Geometry check sheet. Reference: the model listing, model coordinates, mm. Face numbers are marked on the shaded views. A direction names the side the tool comes from. Give positions to 0.01 mm unless a question says otherwise; leave off trailing zeros. Loops run counter-clockwise (first coordinate to the right, second up) from the corner with the lowest first, then second, coordinate; pieces in that order, holes last.
1. Release check for a two-part mould opening along Z. For the marked faces 3, 4, 5 and 6 record: +Z half, -Z half, draft (parallel to the pull), parting line (faces both ways), or undercut.
2. Cross-section at C-C, the plane x = 45. Record the cut outline in (y, z).
3. Tool access check on the marked faces 1 and 2. Record the directions out of +Z, -Z, +X, -X, +Y, -Y that give a thin tool (end or side, any length) a straight path to the whole face; none if there is none.
4. Go/stop test with flat-tipped pins: pin 1 Ø3 at (x, z) = (14.5, -34.5) entering from -Y; pin 2 Ø5 at (x, z) = (0, -21.5) entering from +Y; pin 3 Ø0.8 at (x, z) = (22.5, 21.5) entering from +Y; pin 4 Ø2.5 at (x, z) = (-26, -2.5) entering from +Y. Record where each tip stops, or that it passes through.
5. Cross-section at A-A, the plane y = 10. Record the cut outline in (x, z).
6. Cross-section at D-D, the plane y = 23. Record the cut outline in (x, z), plus the area to 4 significant figures.
7. Material ranges on L1, parallel to X at y = 7.5, z = 0; L2, parallel to Z at x = 33, y = 33.5; L3, parallel to Z at x = -30, y = 29.5, recorded low to high.
8. Cross-section at B-B, the plane x = 31. Record the cut outline in (y, z).
from build123d import *

# Parameters (mm, degrees)
SKETCH1_W               = 87
SKETCH1_H               = 60
HOUSING_DEPTH           = 35
SKETCH4_W               = 82
SKETCH4_H               = 55
HOUSEINTERNALCUT_DEPTH  = 30
SKETCH6_W               = 3.7
SKETCH6_H               = 8.5
SWITCHEXTERNALCUT_DEPTH = 2
SKETCH8_W               = 1.7
SKETCH8_H               = 3.6
SWITCHINTERNALCUT_DEPTH = 4
SKETCH10_R              = 6
BUZZEREXTERNALCUT_DEPTH = 2
SKETCH12_R              = 0.35
BUZZERINTERNALCUT_DEPTH = 4
SKETCH14_W              = 4.6
SKETCH14_H              = 6.1
BUTTONEXTERNALCUT_DEPTH = 2
SKETCH16_R              = 1.5
BUTTONINTERNALCUT_DEPTH = 4
SKETCH29_R              = 17.515
WICHARGECUT_DEPTH       = 3.5
SKETCH30_W              = 59
SKETCH30_H              = 39
RFIDMODULECUT_DEPTH     = 1
SKETCH32_W              = 71
SKETCH32_H              = 25
DISPLAYCUT_DEPTH        = 3.5
MICROUSBCUT_DEPTH       = 2.5
SKETCH34_W              = 6.5
SKETCH34_H              = 3
CLIPSCUT_DEPTH          = 88
SKETCH35_R              = 0.45
RESETCUT_DEPTH          = 6


with BuildPart() as part:
    # Sketch1 → Housing (new body)
    with BuildSketch(Plane(origin=(0, 0, 0), x_dir=(1, 0, 0), z_dir=(0, 1, 0))):
        with Locations((6.529661017, 6.430084746)):
            Rectangle(SKETCH1_W, SKETCH1_H)
    extrude(amount=HOUSING_DEPTH)

    # Sketch4 → HouseInternalCut (cut)
    with BuildSketch(Plane(origin=(0, 35, 0), x_dir=(1, 0, 0), z_dir=(0, 1, 0))):
        with Locations((6.529661017, 6.430084746)):
            Rectangle(SKETCH4_W, SKETCH4_H)
    extrude(amount=-HOUSEINTERNALCUT_DEPTH, mode=Mode.SUBTRACT)

    # Sketch6 → SwitchExternalCut (cut)
    with BuildSketch(Plane(origin=(-29.459679841, 5, 17.678662656), x_dir=(1, 0, 0), z_dir=(0, 1, 0))):
        with Locations((4.354897879, 7.989454328)):
            Rectangle(SKETCH6_W, SKETCH6_H)
    extrude(amount=-SWITCHEXTERNALCUT_DEPTH, mode=Mode.SUBTRACT)

    # Sketch8 → SwitchInternalCut (cut, through all)
    with BuildSketch(Plane(origin=(-29.459679841, 3, 17.678662656), x_dir=(1, 0, 0), z_dir=(0, 1, 0))):
        with Locations((4.354897879, 7.989454328)):
            Rectangle(SKETCH8_W, SKETCH8_H)
    extrude(amount=-SWITCHINTERNALCUT_DEPTH, mode=Mode.SUBTRACT)

    # Sketch10 → BuzzerExternalCut (cut)
    with BuildSketch(Plane(origin=(-0.314920006, 5, -24.188639302), x_dir=(1, 0, 0), z_dir=(0, 1, 0))):
        with Locations((-25.006618322, 0)):
            Circle(SKETCH10_R)
    extrude(amount=-BUZZEREXTERNALCUT_DEPTH, mode=Mode.SUBTRACT)

    # Sketch12 → BuzzerInternalCut (cut, through all)
    with BuildSketch(Plane(origin=(-0.314920006, 3, -24.188639302), x_dir=(1, 0, 0), z_dir=(0, 1, 0))):
        with Locations((-24.042348329, 4.522315504)):
            Circle(SKETCH12_R)
        with Locations((-26.042348329, 3.020429056)):
            Circle(SKETCH12_R)
        with Locations((-28.042348329, 3.020429056)):
            Circle(SKETCH12_R)
        with Locations((-30.042348329, 1.518542609)):
            Circle(SKETCH12_R)
        with Locations((-30.042348329, 0.016656161)):
            Circle(SKETCH12_R)
        with Locations((-30.042348329, -1.485230286)):
            Circle(SKETCH12_R)
        with Locations((-28.042348329, 0.016656161)):
            Circle(SKETCH12_R)
        with Locations((-28.042348329, 1.518542609)):
            Circle(SKETCH12_R)
        with Locations((-28.042348329, -1.485230286)):
            Circle(SKETCH12_R)
        with Locations((-28.042348329, -2.987116733)):
            Circle(SKETCH12_R)
        with Locations((-26.042348329, 0.016656161)):
            Circle(SKETCH12_R)
        with Locations((-26.042348329, 1.518542609)):
            Circle(SKETCH12_R)
        with Locations((-26.042348329, -1.485230286)):
            Circle(SKETCH12_R)
        with Locations((-26.042348329, -2.987116733)):
            Circle(SKETCH12_R)
        with Locations((-26.042348329, -4.489003181)):
            Circle(SKETCH12_R)
        with Locations((-24.042348329, -4.489003181)):
            Circle(SKETCH12_R)
        with Locations((-24.042348329, -2.987116733)):
            Circle(SKETCH12_R)
        with Locations((-24.042348329, -1.485230286)):
            Circle(SKETCH12_R)
        with Locations((-24.042348329, 0.016656161)):
            Circle(SKETCH12_R)
        with Locations((-24.042348329, 1.518542609)):
            Circle(SKETCH12_R)
        with Locations((-24.042348329, 3.020429056)):
            Circle(SKETCH12_R)
        with Locations((-22.042348329, 3.020429056)):
            Circle(SKETCH12_R)
        with Locations((-22.042348329, 1.518542609)):
            Circle(SKETCH12_R)
        with Locations((-22.042348329, 0.016656161)):
            Circle(SKETCH12_R)
        with Locations((-22.042348329, -1.485230286)):
            Circle(SKETCH12_R)
        with Locations((-22.042348329, -2.987116733)):
            Circle(SKETCH12_R)
        with Locations((-20.042348329, -1.485230286)):
            Circle(SKETCH12_R)
        with Locations((-20.042348329, 0.016656161)):
            Circle(SKETCH12_R)
        with Locations((-20.042348329, 1.518542609)):
            Circle(SKETCH12_R)
        with Locations((-26.042348329, 4.522315504)):
            Circle(SKETCH12_R)
    extrude(amount=-BUZZERINTERNALCUT_DEPTH, mode=Mode.SUBTRACT)

    # Sketch14 → ButtonExternalCut (cut)
    with BuildSketch(Plane(origin=(-24.227687265, 5, -14.72402786), x_dir=(1, 0, 0), z_dir=(0, 1, 0))):
        with Locations((-1.096336387, -10.602688636)):
            Rectangle(SKETCH14_W, SKETCH14_H)
    extrude(amount=-BUTTONEXTERNALCUT_DEPTH, mode=Mode.SUBTRACT)

    # Sketch16 → ButtonInternalCut (cut, through all)
    with BuildSketch(Plane(origin=(-24.227687265, 3, -14.72402786), x_dir=(1, 0, 0), z_dir=(0, 1, 0))):
        with Locations((-1.096336387, -10.602688636)):
            Circle(SKETCH16_R)
    extrude(amount=-BUTTONINTERNALCUT_DEPTH, mode=Mode.SUBTRACT)

    # Sketch29 → WiChargeCut (cut)
    with BuildSketch(Plane(origin=(0, 5, 0), x_dir=(1, 0, 0), z_dir=(0, 1, 0))):
        with Locations((6.529661017, 6.430084746)):
            Circle(SKETCH29_R)
    extrude(amount=-WICHARGECUT_DEPTH, mode=Mode.SUBTRACT)

    # Sketch30 → RFIDModuleCut (cut)
    with BuildSketch(Plane(origin=(0, 0, 21.069915254), x_dir=(-1, 0, 0), z_dir=(0, 0, -1))):
        with Locations((-10.029661017, 25.5)):
            Rectangle(SKETCH30_W, SKETCH30_H)
    extrude(amount=-RFIDMODULECUT_DEPTH, mode=Mode.SUBTRACT)

    # Sketch32 → DisplayCut (cut, through all)
    with BuildSketch(Plane.XY.offset(-33.930084746)):
        with Locations((6.529661017, 20.5)):
            Rectangle(SKETCH32_W, SKETCH32_H)
    extrude(amount=-DISPLAYCUT_DEPTH, mode=Mode.SUBTRACT)

    # Sketch33 → MicroUSBCut (cut)
    with BuildSketch(Plane(origin=(50.029661017, 0, 0), x_dir=(0, 0, -1), z_dir=(1, 0, 0))):
        with BuildLine():
            Line((2.705084746, 11), (10.155084746, 11))
            ThreePointArc((10.155084746, 11), (11.155084746, 10), (10.155084746, 9))
            Line((10.155084746, 9), (2.705084746, 9))
            ThreePointArc((2.705084746, 9), (1.705084746, 10), (2.705084746, 11))
        make_face()
    extrude(amount=-MICROUSBCUT_DEPTH, mode=Mode.SUBTRACT)

    # Sketch34 → ClipsCut (cut, through all)
    with BuildSketch(Plane.ZY.offset(36.970338983)):
        with Locations((-22.680084746, 28.64745115)):
            Rectangle(SKETCH34_W, SKETCH34_H)
        with Locations((9.819915254, 28.64745115)):
            Rectangle(SKETCH34_W, SKETCH34_H)
    extrude(amount=-CLIPSCUT_DEPTH, mode=Mode.SUBTRACT)

    # Sketch35 → ResetCut (cut, through all)
    with BuildSketch(Plane(origin=(0, 5, 0), x_dir=(1, 0, 0), z_dir=(0, 1, 0))):
        with Locations((46.529661017, -2.509915254)):
            Circle(SKETCH35_R)
    extrude(amount=-RESETCUT_DEPTH, mode=Mode.SUBTRACT)


solid = part.part
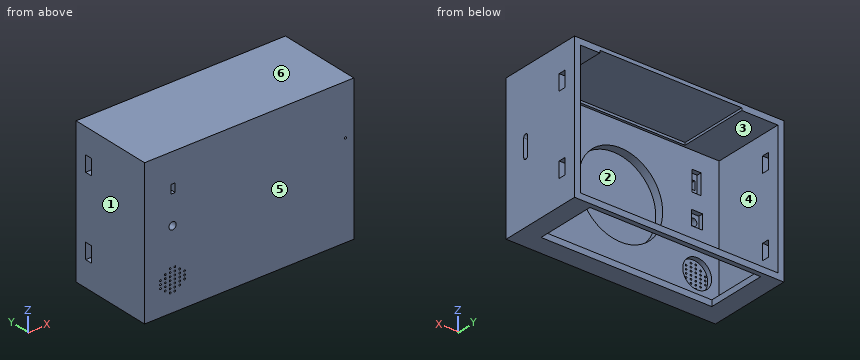
Result:
1. face 3: undercut
1. face 4: undercut
1. face 5: draft
1. face 6: +Z half
2. outline: (0, -36.43) - (35, -36.43) - (35, -33.93) - (5, -33.93) - (5, 21.07) - (35, 21.07) - (35, 23.57) - (0, 23.57) - close
3. face 1: +Z, -Z, -X, +Y, -Y
3. face 2: +Y
4. pin 1: stops at y = 0
4. pin 2: stops at y = 5
4. pin 3: stops at y = 6
4. pin 4: stops at y = 3
5. outline: (-36.97, -36.43) - (-28.97, -36.43) - (-28.97, -33.93) - (-34.47, -33.93) - (-34.47, 21.07) - (-19.47, 21.07) - (-19.47, 22.07) - (39.53, 22.07) - (39.53, 21.07) - (47.53, 21.07) - (47.53, -1.71) - (50.03, -1.71) - (50.03, 23.57) - (-36.97, 23.57) - close; (42.03, -36.43) - (50.03, -36.43) - (50.03, -11.16) - (47.53, -11.16) - (47.53, -33.93) - (42.03, -33.93) - close
6. outline: (-36.97, -36.43) - (-28.97, -36.43) - (-28.97, -33.93) - (-34.47, -33.93) - (-34.47, 21.07) - (-19.47, 21.07) - (-19.47, 22.07) - (39.53, 22.07) - (39.53, 21.07) - (47.53, 21.07) - (47.53, -33.93) - (42.03, -33.93) - (42.03, -36.43) - (50.03, -36.43) - (50.03, 23.57) - (-36.97, 23.57) - close
6. area: 473.5 mm2
7. L1: x = -36.97 to -34.47, 47.53 to 50.03
7. L2: z = -36.43 to -33.93, 22.07 to 23.57
7. L3: z = -36.43 to -33.93, 21.07 to 23.57
8. outline: (0, -36.43) - (8, -36.43) - (8, -33.93) - (5, -33.93) - (5, 21.07) - (6, 21.07) - (6, 22.07) - (35, 22.07) - (35, 23.57) - (0, 23.57) - close; (33, -36.43) - (35, -36.43) - (35, -33.93) - (33, -33.93) - close
